Source: CAD feature listing. Evaluate the final solid. Frame: model axes, mm. Face numbers are marked on the shaded views. Round coordinates to 2 decimals unless told otherwise and drop trailing zeros. Order: outer loops, then holes, each group sorted by start corner. A loop starts at its lowest first (then second) coordinate and runs counter-clockwise, first axis right, second up. Notation, with made-up numbers: (38, -18) -> (54, -18) arc R37 ccw to (54, 19) -> close; hole circle Ø6 at (25, -30.5). An arc over 180 degrees is marked (long way). Answer as CSV lines item,"result". Start each with the question number.
(1) Section query A-A (x = 60). Output: boundary loops of the cut face in (y, z).
(2) Pull-direction query (X, two-part tool) for the marked faces 1 and 2; classes: +X half, -X half, draft (parallel to the pull), parting line (faces both ways), or undercut.
(3) Section query B-B (z = -59.5). Output: boundary loops of the cut face in (x, y).
(4) Contact query for flat-ended pins moving along their axis: P1, Ø12, axis at x = 114, z = 47, coming from the +Y side; P2, Ø4.5, axis at x = 41.5, z = -121, coming from the +Y side; P3, Ø0.8, axis at x = 77.5, y = -0.5, coming from the +Z side. Output: stop coordinate, or through.
(5) Line query: line 1 along Z through (x, y) = (113, 1.35); line 2 along Z through (x, y) = (113, 1.75); line 3 along X through (y, z) = (0.55, 65.5). Output: solid intervals per line, ascending. Write a range as from..to.
```python
from build123d import *

# Parameters (mm, degrees)
SKETCH1_W           = 250
SKETCH1_H           = 250
BOSS_EXTRUDE1_DEPTH = 2.5
SKETCH2_W           = 247
SKETCH2_H           = 247
CUT_EXTRUDE1_DEPTH  = 1
CUT_EXTRUDE4_DEPTH  = 4
CIRPATTERN1_COUNT   = 4
FILLET2_R           = 2
FILLET3_R           = 1


with BuildPart() as part:
    # Sketch1 → Boss-Extrude1 (new, symmetric)
    with BuildSketch(Plane(origin=(0, 0, 0), x_dir=(1, 0, 0), z_dir=(0, 1, 0))):
        Rectangle(SKETCH1_W, SKETCH1_H)
    extrude(amount=BOSS_EXTRUDE1_DEPTH, both=True)

    # Sketch2 → Cut-Extrude1 (cut)
    with BuildSketch(Plane(origin=(0, 2.5, 0), x_dir=(1, 0, 0), z_dir=(0, 1, 0))):
        Rectangle(SKETCH2_W, SKETCH2_H)
    extrude(amount=-CUT_EXTRUDE1_DEPTH, mode=Mode.SUBTRACT)

    # Sketch5 → Cut-Extrude4 (cut)
    with BuildSketch(Plane(origin=(0, 2.5, 0), x_dir=(1, 0, 0), z_dir=(0, 1, 0))):
        Polygon((-75, -125), (-75, -117), (-80, -117), (-80, -110), (-20, -110), (-20, -117), (-25, -117), (-25, -125), align=None)
        with BuildLine():
            Line((25, -125), (75, -125))
            ThreePointArc((75, -125), (80.216117819, -117.5), (75, -110))
            Line((75, -110), (25, -110))
            ThreePointArc((25, -110), (19.783882181, -117.5), (25, -125))
        make_face()
    cut_extrude4 = extrude(amount=-CUT_EXTRUDE4_DEPTH, mode=Mode.SUBTRACT)

    # CirPattern1: Cut-Extrude4 ×4 about axis
    cirpattern1_axis = Axis((0, 0, 0), (0, 1, 0))
    for i in range(1, CIRPATTERN1_COUNT):
        add(cut_extrude4.rotate(cirpattern1_axis, i * 360 / CIRPATTERN1_COUNT), mode=Mode.SUBTRACT)

    # Fillet2
    fillet2_edges = [part.edges().sort_by_distance(p)[0] for p in [
        (-110, 0, 25),
        (-110, 0, 75),
        (-117, 0, -75),
        (-117, 0, -80),
        (-110, 0, -80),
        (-110, 0, -20),
        (-117, 0, -20),
        (-117, 0, -25),
        (-25, 0, -110),
        (-75, 0, -110),
        (123.5, 2, -123.5),
        (75, 0, -117),
        (80, 0, -117),
        (80, 0, -110),
        (123.5, 2, 123.5),
        (20, 0, -110),
        (20, 0, -117),
        (25, 0, -117),
        (-123.5, 2, 123.5),
        (-123.5, 2, -123.5),
        (110, 0, -25),
        (110, 0, -75),
        (117, 0, 75),
        (117, 0, 80),
        (110, 0, 80),
        (110, 0, 20),
        (117, 0, 20),
        (117, 0, 25),
        (-75, 0, 117),
        (-80, 0, 117),
        (-80, 0, 110),
        (-20, 0, 110),
        (-20, 0, 117),
        (-25, 0, 117),
        (25, 0, 110),
        (75, 0, 110),
    ]]
    fillet(fillet2_edges, radius=FILLET2_R)

    # Fillet3
    fillet3_edges = [part.edges().sort_by_distance(p)[0] for p in [
        (-75, 0.5, -125),
        (-25, 0.5, -125),
        (125, 0.5, -25),
        (125, 0.5, -75),
        (25, 0.5, 125),
        (75, 0.5, 125),
        (-125, 0.5, 75),
        (-125, 0.5, 25),
    ]]
    fillet(fillet3_edges, radius=FILLET3_R)


solid = part.part
```
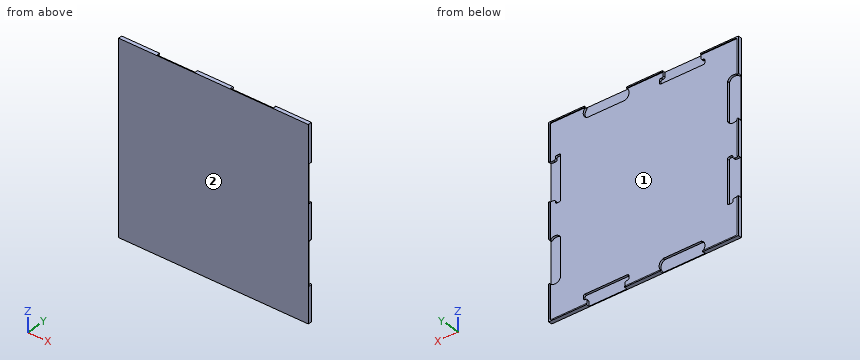
Answer block:
1,outline,"(-2.5, -125) -> (-1.5, -125) -> (-1.5, -110) -> (1.5, -110) -> (1.5, 110) -> (-1.5, 110) -> (-1.5, 125) -> (-2.5, 125) -> close"
2,face 1,"undercut"
2,face 2,"draft"
3,outline,"(-125, -2.5) -> (125, -2.5) -> (125, -1.5) -> (110, -1.5) -> (110, 1.5) -> (-110, 1.5) -> (-110, -1.5) -> (-125, -1.5) -> close"
4,P1,"y = 1.5"
4,P2,"y = -1.5"
4,P3,"z = 124.84"
5,line 1,"-125..-78.83, -21.17..20, 80..125"
5,line 2,"-125..-123.5, 123.5..125"
5,line 3,"-110..110"
